Work out the finished part from the listing and answer in its coordinate system (mm). A direction names the side the tool comes from. Give positions to 0.01 mm unless a question says otherwise; leave off trailing zeros. Write each loop counter-clockwise with the first axis right and the second up, starting at its lowest first coordinate (ties: lowest second). Pieces come first, ordered by that corner, then holes. Notation, with made-up numbers: (81.5, 44.5) -> (97.5, 44.5) arc R19 ccw to (97.5, 71.5) -> close; hole circle Ø2 at (60.5, 13). An arc over 180 degrees is marked (long way). Use a Markdown table: item, result. Add a question column.
Q1. Section B-B, the plane x = -1 is taken. Give the vertices of the cut face in (y, z).
Q2. Section D-D, the plane y = 5.5 is taken. Give the vertices of the cut face in (x, z).
Q3. Each of these flat-tipped pins is pushed along its axis until it touches: pin 1 Ø8 at (x, y) = (-27.5, -15) entering from +Z; pin 2 Ø3.5 at (x, y) = (-88.5, 25) entering from +Z; pin 3 Ø16 at (y, z) = (-6.5, 21.5) entering from +X. Where does it stop, or does it pass through?
Q4. For faces 4 (the face through (-104.083, -24.741, 0.479)), 5 (the face through (-78.44, 0.98, 12.72)), 6 (the face through (-44.5, -3, 11)), 7 (the face through (-67.458, 18, -1)), 8 (the face through (-12, -11, 2)), determine the directions among +Z, -Z, +X, -X, +Y, -Y from which every point of the face is accessible in a straight line to the end or side of a thin tool.
Q5. For a pull along X with two mould halves and no side action, classify faces 1 (the face through (13.9, -20, -1)), 2 (the face through (-86.5, -24.19, -3.03)), 3 (the face through (-7, -9.9, -2)) as pulls with the +X half, pulls with the -X half, needs draft (parallel to the pull), parting line crosses it, or undercut.
Q6. Section C-C, the plane z = 22.5 is taken. Give the vertices of the cut face in (x, y).
Q7. Section A-A, the plane y = 24.5 is taken. Give the vertices of the cut face in (x, z).
Q8. Consider line 1 (Y direction, x = -87.5, z = -3.3); line 2 (X direction, y = -25.5, z = 0.55); line 3 (X direction, y = 24.5, z = 0.15). Determine where each line is inside the solid, lowest interval first.
Autodesk Inventor part; units mm, degrees
ref_plane "Work Plane12" through (-127.4584, -23.859, -5) normal (0, 0, 1) x (1, 0, 0)
ref_plane "Work Plane14" through (-127.4584, -23.859, -5) normal (0, 0, 1) x (1, 0, 0)
ref_plane "YZ Plane" through (0, 0, 0) normal (1, 0, 0) x (0, 1, 0)
ref_plane "Work Plane10" through (-44.5, -14.2241, 18.7548) normal (1, 0, 0) x (0, -0.9087, 0.4175)
ref_plane "Work Plane11" through (-44.5, -8.5, 18.5) normal (-1, 0, 0) x (0, -1, 0)
sketch "Sketch9" plane through (-44.5, -8.5, 18.5) normal (-1, 0, 0) x (0, -1, 0)
  line L0 (16.8555, -12.7) -> (20, -12.7) construction
  circle A0 centre (17.5, -10) radius 1 construction
  circle A1 centre (11, 10.5) radius 1 construction
  circle A2 centre (-10.5, -5) radius 1 construction
  circle A3 centre (0, 0) radius 2.4142 construction
  line L1 (-15, 15) -> (15, 15) construction
  line L2 (16, -16) -> (-16, -16) construction
  line L3 (15, 15) -> (15, -15) construction
  line L4 (16, 16) -> (16, -16) construction
  line L5 (-16, -16) -> (-16, 16) construction
  line L6 (15, 15) -> (-16, 15)
  line L7 (-16, 15) -> (-16, -16.5)
  line L8 (-16, -16.5) -> (15, -16.5)
  line L9 (15, -16.5) -> (15, 15)
  circle A4 centre (11, 10.5) radius 0.9
  circle A5 centre (17.5, -10) radius 0.9
  circle A6 centre (-10.5, -5) radius 0.9
  circle A7 centre (0, 0) radius 9
  line L10 (15, -16.5) -> (22, -16.5)
  line L11 (22, -16.5) -> (22, -7.5)
  line L12 (22, -7.5) -> (15, -7.5)
  line L13 (15, -7.5) -> (15, -16.5)
  point P0 (-8.5, -18.5)
  dimension "d34" = 31.5
  dimension "d35" = 1.8
  dimension "d36" = 1.8
  dimension "d37" = 1.8
  dimension "d38" = 18
  dimension "d39" = 7
  dimension "d40" = 9
extrude "Extrusion7" add sketch "Sketch9" against normal blind 5
ref_plane "Work Plane12" through (-127.4584, -23.859, -5) normal (0, 0, 1) x (1, 0, 0)
sketch "Sketch10" plane through (-44.5, -30.5, 2) normal (0, 0, -1) x (-1, 0, 0)
  line L0 (0, 0) -> (0, 38)
  line L1 (0, 38) -> (-5, 38)
  line L2 (-5, 0) -> (-5, 38)
  line L3 (0, 0) -> (-5, 0)
  circle A0 centre (-19, 22) radius 1.4
  circle A1 centre (-57, 22) radius 1.4
  line L4 (82.9584, 8.641) -> (82.9584, 51.641)
  line L5 (-58.4, 38) -> (82.9584, 38)
  line L6 (82.9584, 38) -> (82.9584, 0)
  line L7 (82.9584, 0) -> (-58.4, 0)
  line L8 (-58.4, 0) -> (-58.4, 38)
  line L9 (-63.3254, 22) -> (-14.2903, 22) construction
  line L10 (-61.7754, 20.45) -> (-15.8403, 20.45)
  line L11 (-15.8403, 23.55) -> (-61.7754, 23.55)
  arc A2 (-61.7754, 23.55) -> (-61.7754, 20.45) centre (-61.7754, 22) ccw
  arc A3 (-15.8403, 20.45) -> (-15.8403, 23.55) centre (-15.8403, 22) ccw
  point P0 (-44.5, 30.5)
  point P1 (-38.8079, 22)
  dimension "d43" = 3.1
extrude "Extrusion8" add sketch "Sketch10" along normal up to surface (7 mm away) contours L3 L2 L1 L0 | L0 L5 L4 L6 L7 | L7 L8 L10 A3 L11 L5 L2 | L8 L11 A3 L10
sketch "Sketch11" plane through (-44.5, -30.5, -5) normal (0, 0, -1) x (-1, 0, 0)
  circle A0 centre (-57, 22) radius 1.4
  circle A1 centre (-19, 22) radius 1.4
  line L0 (-61.4468, 22) -> (-14.0111, 22) construction
  line L1 (-60.0468, 20.6) -> (-15.4111, 20.6)
  line L2 (-15.4111, 23.4) -> (-60.0468, 23.4)
  arc A2 (-60.0468, 23.4) -> (-60.0468, 20.6) centre (-60.0468, 22) ccw
  arc A3 (-15.4111, 20.6) -> (-15.4111, 23.4) centre (-15.4111, 22) ccw
  point P0 (-44.5, 30.5)
  point P1 (-58.4, 22)
  point P2 (-37.729, 22)
extrude "Extrusion9" cut sketch "Sketch11" against normal through all contours A0 | A0 L2 A1 L1 | A0 L1 A2 L2 | L2 A3 L1 A1
ref_plane "Work Plane13" through (-74.5, -8.5, 18.5) normal (-1, 0, 0) x (0, 0, 1)
sketch "Sketch12" plane through (-74.5, -8.5, 18.5) normal (-1, 0, 0) x (0, 0, 1)
  circle A0 centre (0, 0) radius 10.125
  line L0 (-31.5, -12.684) -> (-23.5, -12.684)
  line L1 (-1.4, 6.6) -> (-6.6, 6.6)
  line L2 (-23.5, -22) -> (-23.5, 16)
  line L3 (-16.5, -22) -> (-23.5, -22)
  line L4 (-16.5, 16) -> (-16.5, -22)
  line L5 (-16.5, 16) -> (-23.5, 16)
  line L6 (15, 15) -> (15, -15)
  line L7 (-16.5, -22) -> (15, -22)
  line L8 (15, -22) -> (15, 16)
  line L9 (15, 16) -> (-16.5, 16)
  line L10 (-16.5, 16) -> (-16.5, -22)
  circle A1 centre (0, 0) radius 11.1
  line L11 (11.1, -5.0801) -> (11.1, 4.7426)
  line L12 (-1.1505, -12.1529) -> (-10.0048, -7.0409)
  line L13 (-10.0048, 7.0409) -> (-1.4428, 11.9842)
  arc A2 (-1.1505, -12.1529) -> (11.1, -5.0801) centre (0, 0) ccw
  arc A3 (11.1, 4.7426) -> (-1.4428, 11.9842) centre (0, 0) ccw
  arc A4 (-10.0048, 7.0409) -> (-10.0048, -7.0409) centre (0, 0) ccw
  point P0 (-18.5, 8.5)
  dimension "d51" = 60
  dimension "d52" = 60
  dimension "d73" = 22.2
extrude "Extrusion10" add sketch "Sketch12" along normal blind 8 contours L4 L9 L8 L6 L7
sketch "Sketch13" plane through (-74.5, -30.5, 33.5) normal (0, 0, 1) x (1, 0, 0)
  line L0 (0, 38) -> (0, 0)
  line L1 (0, 38) -> (-8, 38)
  line L2 (-8, 0) -> (-8, 38)
  line L3 (0, 0) -> (-8, 0)
  line L4 (6.7208, 32.125) -> (-12.4892, 32.125)
  circle A0 centre (-4, 22.9829) radius 1.45
  point P0 (74.5, 30.5)
  dimension "d55" = 2.9
extrude "Extrusion11" cut sketch "Sketch13" against normal blind 8 contours A0
sketch "Sketch14" plane through (-44.5, -30.5, 2) normal (0, 0, 1) x (1, 0, 0)
  circle A0 centre (-63, 55) radius 1.45
  circle A1 centre (-43, 55) radius 1.45
  line L0 (-30, 38) -> (-38, 38)
  line L1 (-82.9584, 38) -> (58.4, 38)
  line L2 (-82.9584, 38) -> (-22.9584, 38)
  line L3 (-22.9584, 38) -> (-22.9584, 60)
  line L4 (-22.9584, 60) -> (-82.9584, 60)
  line L5 (-82.9584, 60) -> (-82.9584, 38)
  point P0 (44.5, 30.5)
  dimension "d71" = 60
  dimension "d72" = 22
ref_plane "Work Plane14" through (-127.4584, -23.859, -5) normal (0, 0, 1) x (1, 0, 0)
extrude "Extrusion12" add sketch "Sketch14" against normal up to surface (7 mm away)
sketch "Sketch15" plane through (-44.5, -30.5, 2) normal (0, 0, 1) x (1, 0, 0)
  line L0 (-82.9584, 0) -> (-38, 0)
  line L1 (-38, 0) -> (-38, 38)
  line L2 (-30, 38) -> (-38, 38)
  line L3 (-30, 38) -> (-30, 0)
  line L4 (-30, 0) -> (0, 0)
  line L5 (0, 0) -> (0, 38)
  line L6 (0, 38) -> (-22.9584, 38)
  line L7 (58.4, 20.6) -> (15.4111, 20.6)
  arc A0 (15.4111, 23.4) -> (15.4111, 20.6) centre (15.4111, 22) ccw
  line L8 (15.4111, 23.4) -> (58.4, 23.4)
  line L9 (58.4, 23.4) -> (58.4, 38)
  line L10 (5, 0) -> (5, 38)
  line L11 (5, 0) -> (58.4, 0)
  line L12 (58.4, 0) -> (58.4, 20.6)
  line L13 (-22.9584, 38) -> (-22.9584, 60)
  line L14 (-22.9584, 60) -> (-82.9584, 60)
  circle A1 centre (-63, 5) radius 1.45
  circle A2 centre (-43, 5) radius 1.45
  circle A3 centre (-43, 55) radius 1.45
  circle A4 centre (-63, 55) radius 1.45
  line L15 (-82.9584, 60) -> (-82.9584, 0)
  line L16 (58.4, 38) -> (5, 38)
  point P0 (44.5, 30.5)
  point P1 (-42.9584, 11.641)
  point P2 (-62.9584, 11.641)
hole "Hole3" at (-107.5, -25.5, 2) at (-87.5, -25.5, 2) at (-107.5, 24.5, 2) at (-87.5, 24.5, 2) direction (0, 0, -1) diameter 3.3 end through all counterbore diameter 7 counterbore depth 3
properties part number "cellSTORM_inverted_Laser_left"
Result set:
| question | item | result |
|---|---|---|
| 1 | outline | (-30.5, -5) -> (-9.9, -5) -> (-9.9, 2) -> (-30.5, 2) -> close; (-7.1, -5) -> (7.5, -5) -> (7.5, 2) -> (-7.1, 2) -> close |
| 2 | outline | (-127.46, -5) -> (13.9, -5) -> (13.9, 2) -> (-39.5, 2) -> (-39.5, 33.5) -> (-44.5, 33.5) -> (-44.5, 2) -> (-74.5, 2) -> (-74.5, 33.5) -> (-82.5, 33.5) -> (-82.5, 2) -> (-127.46, 2) -> close |
| 3 | pin 1 | stops at z = 2 |
| 3 | pin 2 | stops at z = -1 |
| 3 | pin 3 | stops at x = -39.5 |
| 4 | face 4 | +Z |
| 4 | face 5 | -X |
| 4 | face 6 | +Z, +Y, -Y |
| 4 | face 7 | +Z, -Z, +X, +Y |
| 4 | face 8 | +Z, +X, +Y, -Y |
| 5 | face 1 | pulls with the +X half |
| 5 | face 2 | undercut |
| 5 | face 3 | needs draft |
| 6 | outline | (-82.5, -30.5) -> (-74.5, -30.5) -> (-74.5, -20.03) -> (-82.5, -20.03) -> close; (-82.5, 2.89) -> (-74.5, 2.89) -> (-74.5, 7.5) -> (-82.5, 7.5) -> close; (-44.5, -23.5) -> (-39.5, -23.5) -> (-39.5, -16.56) -> (-44.5, -16.56) -> close; (-44.5, -0.44) -> (-39.5, -0.44) -> (-39.5, 7.5) -> (-44.5, 7.5) -> close |
| 7 | outline | (-127.46, -5) -> (-109.15, -5) -> (-109.15, -1) -> (-111, -1) -> (-111, 2) -> (-127.46, 2) -> close; (-105.85, -5) -> (-89.15, -5) -> (-89.15, -1) -> (-91, -1) -> (-91, 2) -> (-104, 2) -> (-104, -1) -> (-105.85, -1) -> close; (-85.85, -5) -> (-67.46, -5) -> (-67.46, 2) -> (-84, 2) -> (-84, -1) -> (-85.85, -1) -> close |
| 8 | line 1 | y = -30.5 to -27.15, -23.85 to 22.85, 26.15 to 29.5 |
| 8 | line 2 | x = -127.46 to -111, -104 to -91, -84 to 13.9 |
| 8 | line 3 | x = -127.46 to -111, -104 to -91, -84 to -67.46 |
